Could you check a few things on this drawing? It's one solid part, dimensions in mm from its lowest x, y, z. Coordinates: 2 decimals unless noted, no trailing zeros. Write each loop counter-clockwise with the first axis right and the second up, starting at its lowest first coordinate (ties: lowest second). Pieces come first, ordered by that corner, then holes. Notation, with made-up numbers: M 71.25,-15.75 L 88.25,-15.75 A25 ccw 88.25,-1.75 Z; hole C 71,61 d1. An arc over 180 degrees is marked long. Use a Markdown table: item, result.
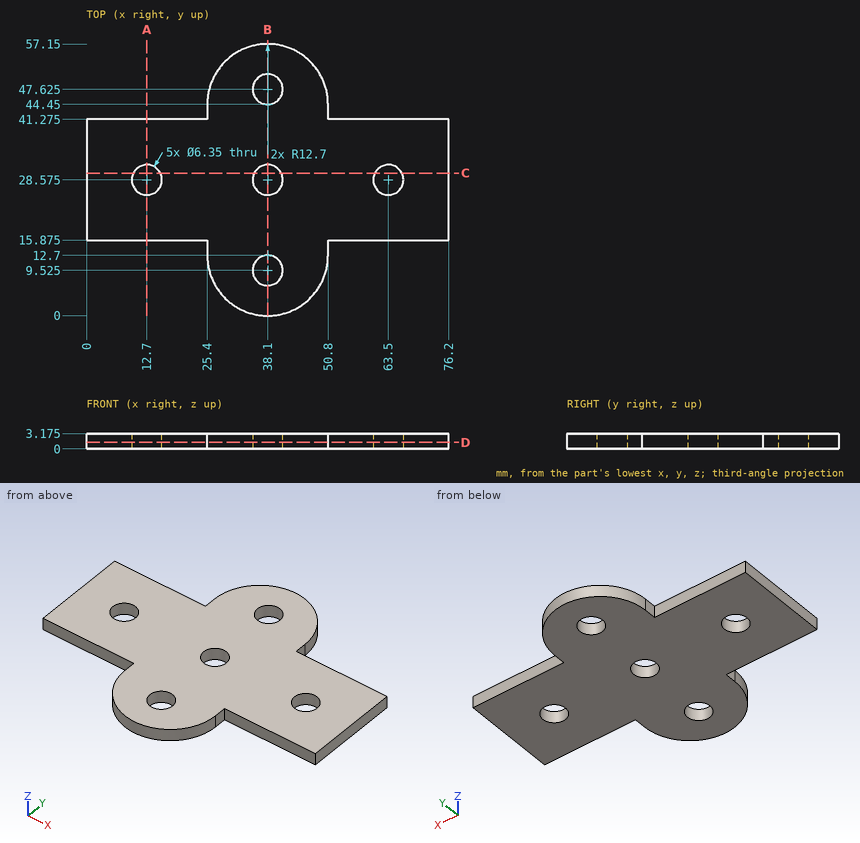
1. Will these pins go through, and if not, where does the flat tip stop? pin 1 Ø1 at (x, z) = (63.5, 2) entering from +Y (3 decimals); pin 2 Ø1.5 at (x, z) = (55, 1) entering from -Y (3 decimals); pin 3 Ø1.6 at (y, z) = (43.5, 1.5) entering from +X; pin 4 Ø4 at (x, y) = (38.1, 9.525) entering from +Z.
Answers follow:
| item | result |
|---|---|
| pin 1 | stops at y = 41.275 |
| pin 2 | stops at y = 15.875 |
| pin 3 | stops at x = 50.8 |
| pin 4 | passes through |
2. Suppose I cut it at A-A on x = 12.7. Write out the boundary of the cut face in (y, z) (3 decimals).
Answers follow:
| item | result |
|---|---|
| outline | M 15.875,0 L 25.4,0 L 25.4,3.175 L 15.875,3.175 Z; M 31.75,0 L 41.275,0 L 41.275,3.175 L 31.75,3.175 Z |
3. Suppose I cut it at B-B on x = 38.1. Write out the boundary of the cut face in (y, z) (3 decimals), and give its area (3 significant figures).
Answers follow:
| item | result |
|---|---|
| outline | M 0,0 L 6.35,0 L 6.35,3.175 L 0,3.175 Z; M 12.7,0 L 25.4,0 L 25.4,3.175 L 12.7,3.175 Z; M 31.75,0 L 44.45,0 L 44.45,3.175 L 31.75,3.175 Z; M 50.8,0 L 57.15,0 L 57.15,3.175 L 50.8,3.175 Z |
| area | 121 mm2 |
4. Suppose I cut it at C-C on y = 30. Write out the boundary of the cut face in (x, z) (3 decimals).
Answers follow:
| item | result |
|---|---|
| outline | M 0,0 L 9.863,0 L 9.863,3.175 L 0,3.175 Z; M 15.537,0 L 35.263,0 L 35.263,3.175 L 15.537,3.175 Z; M 40.937,0 L 60.663,0 L 60.663,3.175 L 40.937,3.175 Z; M 66.337,0 L 76.2,0 L 76.2,3.175 L 66.337,3.175 Z |
5. Suppose I cut it at D-D on z = 1.35. Write out the boundary of the cut face in (x, y) (3 decimals), and give its area (3 significant figures).
Answers follow:
| item | result |
|---|---|
| outline | M 0,15.875 L 25.4,15.875 L 25.4,12.7 A12.7 ccw 50.8,12.7 L 50.8,15.875 L 76.2,15.875 L 76.2,41.275 L 50.8,41.275 L 50.8,44.45 A12.7 ccw 25.4,44.45 L 25.4,41.275 L 0,41.275 Z; hole C 12.7,28.575 d6.35; hole C 38.1,9.525 d6.35; hole C 38.1,28.575 d6.35; hole C 38.1,47.625 d6.35; hole C 63.5,28.575 d6.35 |
| area | 2,450 mm2 |
6. I need wall thicknesses on probe 1 along Y at (x, z) = (38.1, 2.35); probe 2 along Y at (x, z) = (37, 0.3); probe 3 along Y at (x, z) = (63.5, 1.65) (3 decimals). Which ranges of each line are inside material? Lowest first, please.
Answers follow:
| item | result |
|---|---|
| probe 1 | y = 0 to 6.35, 12.7 to 25.4, 31.75 to 44.45, 50.8 to 57.15 |
| probe 2 | y = 0.05 to 6.55, 12.5 to 25.6, 31.55 to 44.65, 50.6 to 57.1 |
| probe 3 | y = 15.875 to 25.4, 31.75 to 41.275 |
